For this review, take the finished solid that the model builds, in its own axes (mm). Face numbers are marked on the shaded views. A direction names the side the tool comes from. Coordinates: 2 decimals unless noted, no trailing zeros. Order: outer loops, then holes, each group sorted by start corner. A loop starts at its lowest first (then second) coordinate and runs counter-clockwise, first axis right, second up.
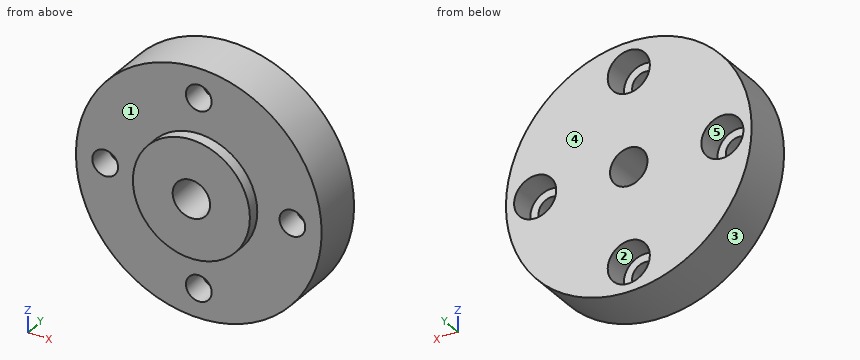
from build123d import *

# Parameters (mm, degrees)
CHAMBRAGE_POUR_VIS_T_TE_CYLINDRIQUE_D           = 11
CHAMBRAGE_POUR_VIS_T_TE_CYLINDRIQUE_CBORE_D     = 18
CHAMBRAGE_POUR_VIS_T_TE_CYLINDRIQUE_CBORE_DEPTH = 11
R_P_TITION_CIRCULAIRE1_COUNT                    = 4


with BuildPart() as part:
    # Esquisse1 → Révolution1 (revolve)
    with BuildSketch(Plane.XY):
        Polygon((8, 0), (8, 27), (52.5, 27), (52.5, 5), (25, 5), (25, 0), align=None)
    revolve(axis=Axis((0, -750.927070457, 0), (0, 1, 0)))

    # Chambrage pour vis à tête cylindrique à 6 pans creux (ou vis CHC) M101 (through all)
    with Locations(Plane(origin=(0, 27, 0), x_dir=(1, 0, 0), z_dir=(0, 1, 0))):
        with Locations((-40, 0)):
            chambrage_pour_vis_t_te_cylindrique = CounterBoreHole(CHAMBRAGE_POUR_VIS_T_TE_CYLINDRIQUE_D / 2, CHAMBRAGE_POUR_VIS_T_TE_CYLINDRIQUE_CBORE_D / 2, CHAMBRAGE_POUR_VIS_T_TE_CYLINDRIQUE_CBORE_DEPTH)

    # Répétition circulaire1: Chambrage pour vis à tête cylindrique à 6 pans creux (ou vis CHC) M101 ×4 about axis
    r_p_tition_circulaire1_axis = Axis((0, 0, 0), (0, 1, 0))
    for i in range(1, R_P_TITION_CIRCULAIRE1_COUNT):
        add(chambrage_pour_vis_t_te_cylindrique.rotate(r_p_tition_circulaire1_axis, i * 360 / R_P_TITION_CIRCULAIRE1_COUNT), mode=Mode.SUBTRACT)


solid = part.part
1. Clearance check with flat-ended pins moving along their axes: pin 1 Ø14.5 at (x, z) = (0.5, 39) entering from +Y; pin 2 Ø20.5 at (x, z) = (0, -40) entering from -Y; pin 3 Ø2 at (y, z) = (19, -23) entering from -X; pin 4 Ø10 at (x, z) = (-37.5, 39.5) entering from +Y. State where each tip first meets the part, or that it passes through.
Answer below:
pin 1: stops at y = 16
pin 2: stops at y = 5
pin 3: stops at x = -47.67
pin 4: stops at y = 27
2. The part is to be moulded in two halves that separate along Z. For the marked faces 1, 2 and 3, say which applies: +Z half, -Z half, draft (parallel to the pull), parting line (faces both ways), or undercut.
Answer below:
face 1: draft
face 2: undercut
face 3: parting line
3. Take a section at C-C, the plane y = 21.75. Give the boundary of the cut face in (x, z), plus the area to 3 significant figures.
Answer below:
outline: circle Ø105 at (0, 0); hole circle Ø18 at (-40, 0); hole circle Ø18 at (0, -40); hole circle Ø18 at (0, 40); hole circle Ø16 at (0, 0); hole circle Ø18 at (40, 0)
area: 7,440 mm2
4. Take a section at B-B, the plane z = 0. Give the boundary of the cut face in (x, y), plus the area to 3 significant figures.
Answer below:
outline: (-52.5, 5) - (-45.5, 5) - (-45.5, 16) - (-49, 16) - (-49, 27) - (-52.5, 27) - close; (-34.5, 5) - (-25, 5) - (-25, 0) - (-8, 0) - (-8, 27) - (-31, 27) - (-31, 16) - (-34.5, 16) - close; (8, 0) - (25, 0) - (25, 5) - (34.5, 5) - (34.5, 16) - (31, 16) - (31, 27) - (8, 27) - close; (45.5, 5) - (52.5, 5) - (52.5, 27) - (49, 27) - (49, 16) - (45.5, 16) - close
area: 1,490 mm2
5. To check wall thickness, follow L1, parallel to Y at x = -4.5, z = 28; L2, parallel to Z at x = -7, y = 21.5; L3, parallel to Z at x = -40.5, y = 21.5. State the ranges of each line that lie inside material, in increasing order.
Answer below:
L1: y = 5 to 27
L2: z = -52.03 to -45.66, -34.34 to -3.87, 3.87 to 34.34, 45.66 to 52.03
L3: z = -33.41 to -8.99, 8.99 to 33.41
6. Take a section at A-A, the plane x = 0. Give the boundary of the cut face in (y, z).
Answer below:
outline: (0, -25) - (5, -25) - (5, -34.5) - (16, -34.5) - (16, -31) - (27, -31) - (27, -8) - (0, -8) - close; (0, 8) - (27, 8) - (27, 31) - (16, 31) - (16, 34.5) - (5, 34.5) - (5, 25) - (0, 25) - close; (5, -52.5) - (27, -52.5) - (27, -49) - (16, -49) - (16, -45.5) - (5, -45.5) - close; (5, 45.5) - (16, 45.5) - (16, 49) - (27, 49) - (27, 52.5) - (5, 52.5) - close
7. Take a section at D-D, the plane x = 44. Give the boundary of the cut face in (y, z), plus the area to 4 significant figures.
Answer below:
outline: (5, -28.64) - (27, -28.64) - (27, -8.06) - (16, -8.06) - (16, -3.77) - (5, -3.77) - close; (5, 3.77) - (16, 3.77) - (16, 8.06) - (27, 8.06) - (27, 28.64) - (5, 28.64) - close
area: 1,000 mm2
8. Machinability: for the marked faces 4 and 5, which of the approach directions +Z, -Z, +X, -X, +Y, -Y give a long, thin tool a straight path to every point of the face, cutting with its end or side? Answer none if there is none.
Answer below:
face 4: +Z, -Z, +X, -X, +Y
face 5: +Y
